```python
from build123d import *

# Parameters (mm, degrees)
CROQUIS1_W              = 18
CROQUIS1_H              = 18
SALIENTE_EXTRUIR1_DEPTH = 10
CROQUIS2_R              = 6.9
CORTAR_EXTRUIR1_DEPTH   = 8
CROQUIS3_R              = 2.75
CORTAR_EXTRUIR2_DEPTH   = 8


with BuildPart() as part:
    # Croquis1 → Saliente-Extruir1 (new body)
    with BuildSketch(Plane.XY):
        Rectangle(CROQUIS1_W, CROQUIS1_H)
    extrude(amount=SALIENTE_EXTRUIR1_DEPTH)

    # Croquis2 → Cortar-Extruir1 (cut)
    with BuildSketch(Plane.XY.offset(10)):
        Circle(CROQUIS2_R)
    extrude(amount=-CORTAR_EXTRUIR1_DEPTH, mode=Mode.SUBTRACT)

    # Croquis3 → Cortar-Extruir2 (cut)
    with BuildSketch(Plane.XY.offset(2)):
        Circle(CROQUIS3_R)
    extrude(amount=-CORTAR_EXTRUIR2_DEPTH, mode=Mode.SUBTRACT)


solid = part.part
```
Part model, mm, in its own coordinate system. A direction names the side the tool comes from. Give positions to 0.01 mm unless a question says otherwise; leave off trailing zeros. Write each loop counter-clockwise with the first axis right and the second up, starting at its lowest first coordinate (ties: lowest second). Pieces come first, ordered by that corner, then holes. Notation, with made-up numbers: (74.25, 67.5) -> (132.25, 67.5) arc R24 ccw to (132.25, 82.5) -> close; hole circle Ø8 at (48, 11). An arc over 180 degrees is marked (long way). Put each result on its own line as item: value. Start each with the question number.
Item 1: Pull direction X, two halves, no side cores. Call faces 3 (the face through (-0.9, 6.84, 6.06)), 4 (the face through (0, 9, 5)), 5 (the face through (9, 0, 5)), 6 (the face through (-0.596, -2.685, 1.014)): pulls with the +X half, pulls with the -X half, needs draft (parallel to the pull), parting line crosses it, or undercut.
Item 2: Cut at C-C (z = 2.5). List the corners of the cut face in (x, y), then the cut area to 3 significant figures.
Item 3: Wall check: L1, parallel to Y at x = 0, z = 7; L2, parallel to Y at x = 0, z = 0.9; L3, parallel to Z at x = -1, y = 3.5. Give the ranges that are in metal, low to high. Write a range as [from, to].
Item 4: Pin check, flat tip, straight feed: pin 1 Ø5 at (x, y) = (0, 2) entering from +Z. Stop position of the tip, or through.
Item 5: Which spindle directions (+Z, -Z, +X, -X, +Y, -Y) get a long thin tool onto all of the face, cutting with end or side? Do faces 1 (the face through (-2.1, 2.1, 0)), 2 (the face through (3, 0, 2)). Say none if no direction does.
Item 6: Cut at D-D (y = -4.75). List the corners of the cut face in (x, z), then the cut area to 3 significant figures.
Item 7: Cut at A-A (y = 0). List the corners of the cut face in (x, z), then the cut area to 3 significant figures.
Answer list:
1. face 3: undercut
1. face 4: needs draft
1. face 5: pulls with the +X half
1. face 6: undercut
2. outline: (-9, -9) -> (9, -9) -> (9, 9) -> (-9, 9) -> close; hole circle Ø13.8 at (0, 0)
2. area: 174 mm2
3. L1: y = [-9, -6.9], [6.9, 9]
3. L2: y = [-9, -2.75], [2.75, 9]
3. L3: z = [0, 2]
4. pin 1: stops at z = 2
5. face 1: -Z, +X, -X, +Y, -Y
5. face 2: +Z
6. outline: (-9, 0) -> (9, 0) -> (9, 10) -> (5, 10) -> (5, 2) -> (-5, 2) -> (-5, 10) -> (-9, 10) -> close
6. area: 99.9 mm2
7. outline: (-9, 0) -> (-2.75, 0) -> (-2.75, 2) -> (-6.9, 2) -> (-6.9, 10) -> (-9, 10) -> close; (2.75, 0) -> (9, 0) -> (9, 10) -> (6.9, 10) -> (6.9, 2) -> (2.75, 2) -> close
7. area: 58.6 mm2
